```python
from build123d import *

# Parameters (mm, degrees)
SKETCH1_W           = 7
SKETCH1_H           = 7
BOSS_EXTRUDE1_DEPTH = 1.53
SKETCH2_R           = 2.54
BOSS_EXTRUDE2_DEPTH = 7.874
SKETCH3_R           = 0.635
BOSS_EXTRUDE3_DEPTH = 3.81
CHAMFER1_SIZE       = 0.25
BOSS_EXTRUDE4_DEPTH = 0.381
SKETCH5_W           = 1.0414
SKETCH5_H           = 1.0414
BOSS_EXTRUDE5_DEPTH = 3.81
SKETCH6_R           = 3
SKETCH6_R_2         = 2.55
FILE_TO_FIT_DEPTH   = 4.191


with BuildPart() as part:
    # Sketch1 → Boss-Extrude1 (new body)
    with BuildSketch(Plane(origin=(0, 0, 0), x_dir=(1, 0, 0), z_dir=(0, 1, 0))):
        Rectangle(SKETCH1_W, SKETCH1_H)
    extrude(amount=BOSS_EXTRUDE1_DEPTH)

    # Sketch2 → Boss-Extrude2 (add)
    with BuildSketch(Plane.XZ):
        with Locations(Location((0, 0, 0), (0, 0, 270))):
            Circle(SKETCH2_R)
    extrude(amount=BOSS_EXTRUDE2_DEPTH)

    # Sketch3 → Boss-Extrude3 (add)
    with BuildSketch(Plane(origin=(0, 1.53, 0), x_dir=(1, 0, 0), z_dir=(0, 1, 0))):
        with Locations(Location((0, 0, 0), (0, 0, 90))):
            Circle(SKETCH3_R)
    extrude(amount=BOSS_EXTRUDE3_DEPTH)

    # Chamfer1
    chamfer1_edges = [part.edges().sort_by_distance(p)[0] for p in [
        (3.5, 0.765, 3.5),
        (-3.5, 0.765, 3.5),
        (-3.5, 0.765, -3.5),
        (3.5, 0.765, -3.5),
    ]]
    chamfer(chamfer1_edges, length=CHAMFER1_SIZE)

    # Sketch4 → Boss-Extrude4 (add)
    with BuildSketch(Plane(origin=(0, 1.53, 0), x_dir=(1, 0, 0), z_dir=(0, 1, 0))):
        Polygon((-3.5, 2), (-2, 2), (-2, 3.5), (-3.25, 3.5), (-3.5, 3.25), align=None)
        Polygon((3.5, 3.25), (3.5, 2), (2, 2), (2, 3.5), (3.25, 3.5), align=None)
        Polygon((3.5, -2), (2, -2), (2, -3.5), (3.25, -3.5), (3.5, -3.25), align=None)
        Polygon((-3.5, -3.25), (-3.5, -2), (-2, -2), (-2, -3.5), (-3.25, -3.5), align=None)
    extrude(amount=BOSS_EXTRUDE4_DEPTH)

    # Sketch5 → Boss-Extrude5 (add)
    with BuildSketch(Plane(origin=(0, 1.911, 0), x_dir=(1, 0, 0), z_dir=(0, 1, 0))):
        with Locations((-2.5207, 2.5207)):
            Rectangle(SKETCH5_W, SKETCH5_H)
        with Locations((2.5207, 2.5207)):
            Rectangle(SKETCH5_W, SKETCH5_H)
        with Locations((2.5207, -2.5207)):
            Rectangle(SKETCH5_W, SKETCH5_H)
        with Locations((-2.5207, -2.5207)):
            Rectangle(SKETCH5_W, SKETCH5_H)
    extrude(amount=BOSS_EXTRUDE5_DEPTH)

    # Sketch6 → File To Fit (cut)
    with BuildSketch(Plane(origin=(0, 5.721, 0), x_dir=(1, 0, 0), z_dir=(0, 1, 0))):
        Circle(SKETCH6_R)
        Circle(SKETCH6_R_2, mode=Mode.SUBTRACT)
    extrude(amount=-FILE_TO_FIT_DEPTH, mode=Mode.SUBTRACT)


solid = part.part
```
Source: CAD feature listing. Evaluate the final solid. Frame: model axes, mm. A direction names the side the tool comes from. Coordinates: 2 decimals unless noted, no trailing zeros. Write each loop counter-clockwise with the first axis right and the second up, starting at its lowest first coordinate (ties: lowest second). Pieces come first, ordered by that corner, then holes. Notation, with made-up numbers: (6, 83.5) -> (12, 83.5) arc R20 cw to (12, 116.5) -> close; hole circle Ø1 at (-20.75, 57). An arc over 180 degrees is marked (long way). Return JSON: item names as keys, results as strings. Group by question number.
1) Section query C-C, the plane x = 0. Return loops of the section in (y, z) (3 decimals).
2) Ray query, line 1 along Y through (x, z) = (0, -0.5); line 2 along Y through (x, z) = (-0.5, -0.5); line 3 along X through (y, z) = (5, 2.75). Return the intervals inside material, ascending.
3) Section query D-D, the plane y = -6.75. Return loops of the section in (x, z).
4) Contact query for flat-ended pins moving along their axis: P1, Ø0.6, axis at y = 3.5, z = -3, coming from the +X side; P2, Ø3, axis at x = -2, y = -2, coming from the +Z side; P3, Ø1, axis at x = 2.5, y = 3, coming from the -Z side. Output: stop coordinate, or through.
5) Set-up query: faces 4 (the face through (-3.041, 3.8, -2.5)), 5 (the face through (2.5, 3.8, -3.041)), 6 (the face through (-2.5, 3.8, 3.041)), 7 (the face through (-0.63, 3.41, 0.08)), 8 (the face through (2, 3.6, -2.7)). Return all of +Z, -Z, +X, -X, +Y, -Y with unobstructed straight access to the full face (end or side cutting, diameter ignored); none if empty.
6) Mould query, pull axis X, two halves, no side actions, for faces 1 (the face through (-2, 3.6, -2.7)), 2 (the face through (-3.041, 3.8, 2.5)), 3 (the face through (2.9, 1.911, 3.2)). Classes: +X half, -X half, draft (parallel to the pull), parting line (faces both ways), or undercut.
7) Section query B-B, the plane z = 0. Return loops of the section in (x, y) (3 decimals).
8) Section query A-A, the plane y = 3.5. Return loops of the section in (x, z) (3 decimals), plus the area to 3 significant figures.
From the geometry:
{
 "1": {"outline": "(-7.874, -2.54) -> (0, -2.54) -> (0, -3.5) -> (1.53, -3.5) -> (1.53, -0.635) -> (5.34, -0.635) -> (5.34, 0.635) -> (1.53, 0.635) -> (1.53, 3.5) -> (0, 3.5) -> (0, 2.54) -> (-7.874, 2.54) -> close"},
 "2": {"line 1": "-7.87 to 5.34", "line 2": "-7.87 to 1.53", "line 3": "-3.04 to -2, 2 to 3.04"},
 "3": {"outline": "circle Ø5.08 at (0, 0)"},
 "4": {"P1": "x = 3.04", "P2": "z = 2.49", "P3": "z = -3.04"},
 "5": {"face 4": "+Z, -Z, -X, +Y", "face 5": "-Z, +X, -X, +Y", "face 6": "+Z, +X, -X, +Y", "face 7": "+Y", "face 8": "+Z, -Z, +Y"},
 "6": {"face 1": "undercut", "face 2": "-X half", "face 3": "draft"},
 "7": {"outline": "(-3.5, 0) -> (-2.54, 0) -> (-2.54, -7.874) -> (2.54, -7.874) -> (2.54, 0) -> (3.5, 0) -> (3.5, 1.53) -> (0.635, 1.53) -> (0.635, 5.34) -> (-0.635, 5.34) -> (-0.635, 1.53) -> (-3.5, 1.53) -> close"},
 "8": {"outline": "(-3.041, -3.041) -> (-2, -3.041) -> (-2, -2.236) arc R3 cw to (-2.236, -2) -> (-3.041, -2) -> close; (-3.041, 2) -> (-2.236, 2) arc R3 cw to (-2, 2.236) -> (-2, 3.041) -> (-3.041, 3.041) -> close; circle Ø1.27 at (0, 0); (2, -3.041) -> (3.041, -3.041) -> (3.041, -2) -> (2.236, -2) arc R3 cw to (2, -2.236) -> close; (2, 2.236) arc R3 cw to (2.236, 2) -> (3.041, 2) -> (3.041, 3.041) -> (2, 3.041) -> close", "area": "5.49 mm²"}
}
